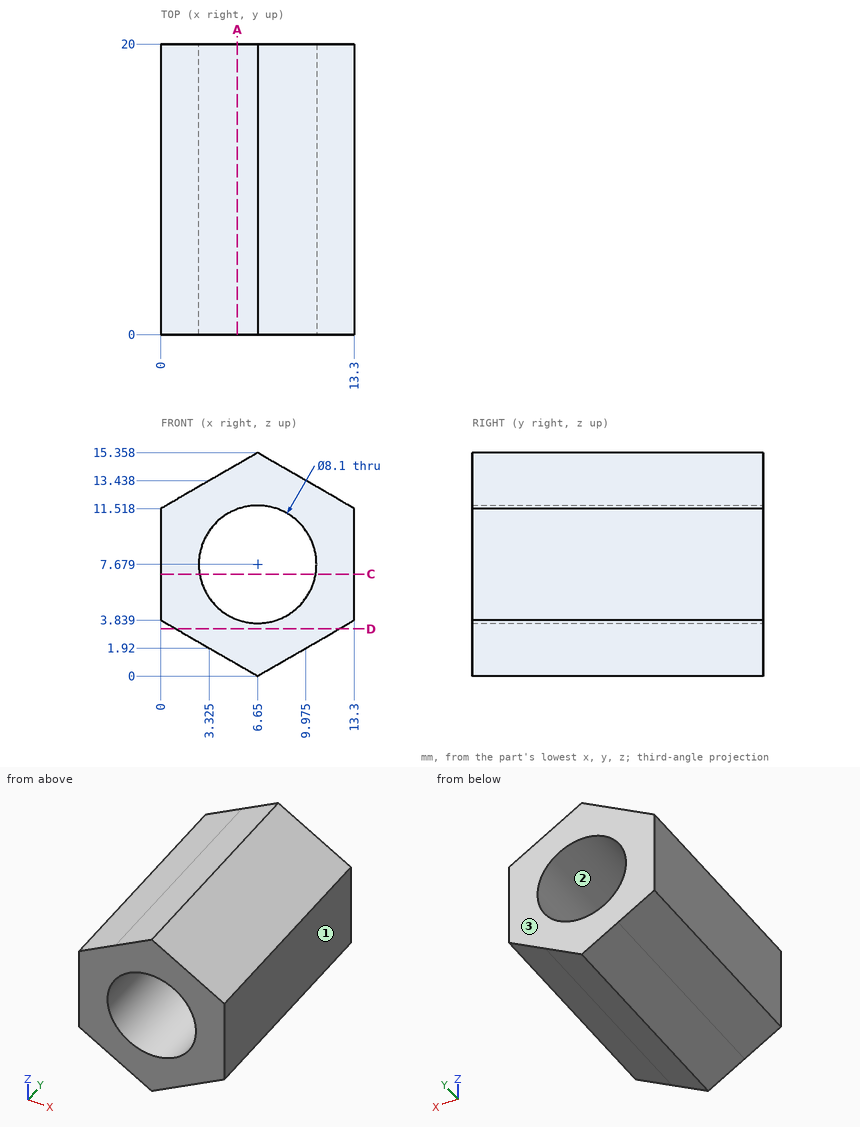
Job drawing, mm, ordinate dimensions from the low corner. One solid piece. Give positions to 0.01 mm unless a question says otherwise; leave off trailing zeros. Loops run counter-clockwise (first coordinate to the right, second up) from the corner with the lowest first, then second, coordinate; pieces in that order, holes last.
Item 1: Drill centre lines: line 1 (X direction, y = 3, z = 5.75); line 2 (X direction, y = 17.5, z = 6.75); line 3 (Z direction, x = 8.5, y = 10.25) (1 decimal). Where is each one in solid material? Low to high.
Answers follow:
line 1: x = 0 to 3.09, 10.21 to 13.3
line 2: x = 0 to 2.71, 10.59 to 13.3
line 3: z = 1.1 to 4.1, 11.3 to 14.3
Item 2: Slice it at C-C, the plane z = 7. List the corners of the cut face in (x, y), and give its area (3 significant figures).
Answers follow:
outline: (0, 0) - (2.66, 0) - (2.66, 20) - (0, 20) - close; (10.64, 0) - (13.3, 0) - (13.3, 20) - (10.64, 20) - close
area: 106 mm2
Item 3: Slice it at A-A, the plane x = 5.25. List the corners of the cut face in (y, z), and give its area (3 significant figures).
Answers follow:
outline: (0, 0.81) - (20, 0.81) - (20, 3.88) - (0, 3.88) - close; (0, 11.48) - (20, 11.48) - (20, 14.55) - (0, 14.55) - close
area: 123 mm2
Item 4: Slice it at D-D, the plane z = 3.25. List the corners of the cut face in (x, y).
Answers follow:
outline: (1.02, 0) - (12.28, 0) - (12.28, 20) - (1.02, 20) - close
Item 5: Flat gauge pin, fed straight in: pin 1 (1.5 mm diameter, centred on x = 5.5, y = 3.5, fed in from +Z). Where does the tip first touch, or does it go through?
Answers follow:
pin 1: stops at z = 15.13
Item 6: Pull direction X, two halves, no side cores. Call the marked faces 1, 2 and 3: released by +X, released by -X, zero draft, split by the parting line, or undercut.
Answers follow:
face 1: released by +X
face 2: undercut
face 3: zero draft
